Autodesk Inventor part; units mm, degrees
ref_plane "YZ Plane" through (0, 0, 0) normal (1, 0, 0) x (0, 1, 0)
ref_plane "XZ Plane" through (0, 0, 0) normal (0, 1, 0) x (-1, 0, 0)
ref_plane "XY Plane" through (0, 0, 0) normal (0, 0, 1) x (1, 0, 0)
sketch "Sketch1" plane through (0, 0, 0) normal (0, 0, 1) x (1, 0, 0)
  line L0 (76.2, -25.4) -> (-76.2, -25.4)
  line L1 (-76.2, -25.4) -> (-76.2, 25.4)
  line L2 (-76.2, 25.4) -> (76.2, 25.4)
  line L3 (76.2, 25.4) -> (76.2, -25.4)
  line L4 (76.2, -25.4) -> (-76.2, 25.4) construction
  line L5 (-76.2, -25.4) -> (76.2, 25.4) construction
  point P0 (0, 0)
  dimension "d0" = 50.8
  dimension "d1" = 152.4
extrude "Extrusion1" add sketch "Sketch1" along normal blind 19.05
sketch "Sketch2" plane through (0, 0, 19.05) normal (0, 0, 1) x (1, 0, 0)
  line L0 (76.2, 25.4) -> (-76.2, 25.4)
  line L1 (-76.2, 25.4) -> (-76.2, -25.4)
  circle A0 centre (-19.05, -26.67) radius 32.258
  line L2 (-76.2, -25.4) -> (76.2, -25.4)
  point P0 (0, 0)
  dimension "d15" = 1.27
  dimension "d16" = 64.516
  dimension "d40" = 57.15
extrude "Extrusion2" cut sketch "Sketch2" against normal through all
sketch "Sketch3" plane through (-76.2, 25.4, 0) normal (0, 1, 0) x (1, 0, 0)
  circle A0 centre (15.875, -9.525) radius 2.5527
  line L0 (152.4, 0) -> (0, 0)
  circle A1 centre (98.425, -9.525) radius 2.5527
  line L1 (57.15, -22.86) -> (57.15, 3.81)
  dimension "d19" = 5.1054
  dimension "d20" = 9.525
  dimension "d24" = 82.55
  dimension "d41" = 41.275
extrude "Extrusion3" cut sketch "Sketch3" against normal through all
sketch "Sketch4" plane through (0, 0, 19.05) normal (0, 0, 1) x (1, 0, 0)
  circle A0 centre (-45.9908, 0.2708) radius 2.5797
  arc A1 (13.183, -25.4) -> (-51.283, -25.4) centre (-19.05, -26.67) ccw
  circle A2 centre (-19.05, 11.43) radius 2.5797
  circle A3 centre (7.8908, 0.2708) radius 2.5797
  line L0 (-19.05, -26.67) -> (-19.05, -17.7805)
  dimension "d31" = 5.1594
  dimension "d32" = 38.1
  dimension "d36" = 90
  dimension "d42" = 45
extrude "Extrusion4" cut sketch "Sketch4" against normal through all
sketch "Sketch5" plane through (0, 0, 19.05) normal (0, 0, 1) x (1, 0, 0)
  circle A0 centre (-69.85, -19.05) radius 3.3734
  arc A1 (13.183, -25.4) -> (-51.283, -25.4) centre (-19.05, -26.67) ccw
  line L0 (-76.2, -25.4) -> (-51.283, -25.4)
  line L1 (-76.2, 25.4) -> (-76.2, -25.4)
  circle A2 centre (-69.85, 19.05) radius 3.3734
  circle A3 centre (31.75, -19.05) radius 3.3734
  circle A4 centre (31.75, 19.05) radius 3.3734
  circle A5 centre (41.611, 17.7518) radius 3.3734
  circle A6 centre (50.8, 13.9456) radius 3.3734
  circle A7 centre (58.6908, 7.8908) radius 3.3734
  circle A8 centre (64.7456, 0) radius 3.3734
  circle A9 centre (68.5518, -9.189) radius 3.3734
  circle A10 centre (69.85, -19.05) radius 3.3734
  point P0 (0, 0)
  dimension "d43" = 6.7469
  dimension "d44" = 50.8
  dimension "d45" = 6.35
  dimension "d55" = 38.1
  dimension "d58" = 101.6
  dimension "d63" = 90
extrude "Extrusion5" cut sketch "Sketch5" against normal through all
equation "\"d24\" = 2 * d41"
equation "\"d58\" = 2 * d44"
properties part number "ShooterSeperableClampB"
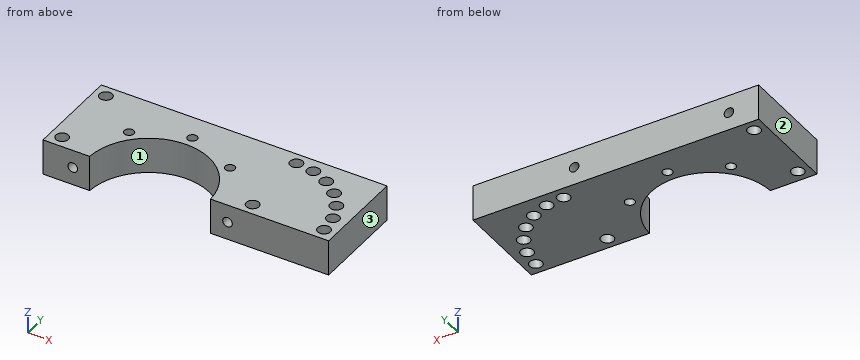
Verification items for the finished model (mm, model axes). Face numbers are marked on the shaded views. Coordinates: 2 decimals unless noted, no trailing zeros. Order: outer loops, then holes, each group sorted by start corner. A loop starts at its lowest first (then second) coordinate and runs counter-clockwise, first axis right, second up. Notation, with made-up numbers: M -40,51.25 L -27,51.25 A21 cw -27,70.25 Z; hole C 15,25.5 d9. An arc over 180 degrees is marked long. One line per item, written item: value. Start each with the question number.
Item 1: Sectioned sample at A-A on y = -19.05. Record the cut outline in (x, z) (3 decimals), then the cut area to 3 significant figures.
Item 2: Mould release check, pull along X, two halves, no side actions. Record for the marked faces 1, 2 and 3: pulls with the +X half, pulls with the -X half, needs draft (parallel to the pull), parting line crosses it, or undercut.
Item 3: Sectioned sample at B-B on x = -69.85. Record the cut outline in (y, z).
Item 4: Thickness scan on probe 1 along Y at (x, z) = (50.8, 14.25); probe 2 along X at (y, z) = (13, 5); probe 3 along X at (y, z) = (-11, 8.5). Record the ranges inside material, lowest first.
Item 5: Sectioned sample at D-D on y = 19.05. Record the cut outline in (x, z) (3 decimals), then the cut area to 3 significant figures.
Item 6: Sectioned sample at C-C on x = -19.05. Record the cut outline in (y, z).
Item 7: Depth check by flat-ended pin: P1, Ø6, axis at x = 6.5, z = 10, coming from the -Y side. Enter the tip coordinate at first touch or a pass-through.
Calculated:
1. outline: M -76.2,0 L -73.223,0 L -73.223,19.05 L -76.2,19.05 Z; M -66.477,0 L -50.395,0 L -50.395,19.05 L -66.477,19.05 Z; M 12.295,0 L 28.377,0 L 28.377,19.05 L 12.295,19.05 Z; M 35.123,0 L 66.477,0 L 66.477,19.05 L 35.123,19.05 Z; M 73.223,0 L 76.2,0 L 76.2,19.05 L 73.223,19.05 Z; hole C -60.325,9.525 d5.105; hole C 22.225,9.525 d5.105
1. area: 1,280 mm^2
2. face 1: undercut
2. face 2: pulls with the -X half
2. face 3: pulls with the +X half
3. outline: M -25.4,0 L -22.42,0 L -22.42,19.05 L -25.4,19.05 Z; M -15.68,0 L 15.68,0 L 15.68,19.05 L -15.68,19.05 Z; M 22.42,0 L 25.4,0 L 25.4,19.05 L 22.42,19.05 Z
4. probe 1: -25.4 to 10.57, 17.32 to 25.4
4. probe 2: -76.2 to -21.1, -17 to 47.56, 54.04 to 76.2
4. probe 3: -76.2 to -62.66, -57.99 to -47.25, 9.15 to 19.89, 24.56 to 65.71, 71.4 to 76.2
5. outline: M -76.2,0 L -73.223,0 L -73.223,19.05 L -76.2,19.05 Z; M -66.477,0 L 28.377,0 L 28.377,19.05 L -66.477,19.05 Z; M 35.123,0 L 38.497,0 L 38.497,19.05 L 35.123,19.05 Z; M 44.725,0 L 76.2,0 L 76.2,19.05 L 44.725,19.05 Z; hole C -60.325,9.525 d5.105; hole C 22.225,9.525 d5.105
5. area: 2,490 mm^2
6. outline: M 5.59,0 L 8.85,0 L 8.85,19.05 L 5.59,19.05 Z; M 14.01,0 L 25.4,0 L 25.4,19.05 L 14.01,19.05 Z
7. P1: y = -11.65
